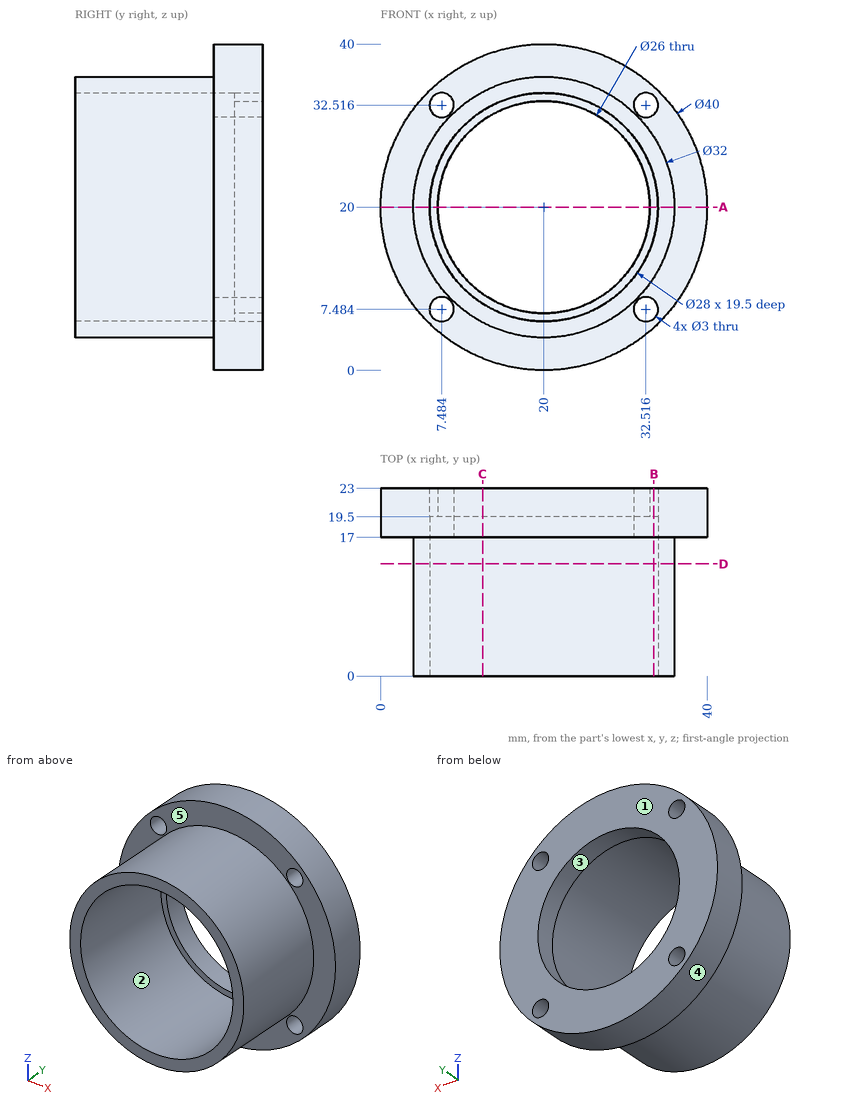
Drawing for the job (mm, zero at the part's lowest x, y, z). A direction names the side the tool comes from. Give positions to 0.01 mm unless a question says otherwise; leave off trailing zeros. Order: outer loops, then holes, each group sorted by start corner. A loop starts at its lowest first (then second) coordinate and runs counter-clockwise, first axis right, second up. Notation, with made-up numbers: (-30.75, 39.5) - (5.25, 39.5) arc R22 ccw to (5.25, 69.5) - close; hole circle Ø3 at (-5, 2.5). An arc over 180 degrees is marked (long way). Use one line per item in the form item = value.
Item 1: Probe probe 1 along X at (y, z) = (22.15, 20); probe 2 along X at (y, z) = (8.25, 20); probe 3 along Y at (x, z) = (24, 32.5). List the from-to ranges inside material, lowest first. Write a range as from..to.
Solution:
probe_1 = 0..7, 33..40
probe_2 = 4..6, 34..36
probe_3 = 19.5..23
Item 2: Pin check, flat tips, straight feed: pin 1 Ø10 at (x, y) = (17, 12.5) entering from -Z; pin 2 Ø17 at (x, z) = (20, 20) entering from -Y; pin 3 Ø4 at (x, z) = (31, 26) entering from -Y; pin 4 Ø14 at (x, z) = (17.5, 13.5) entering from -Y. Stop position of each tip, or through.
Solution:
pin_1 = 0.02
pin_2 = through
pin_3 = 0
pin_4 = 19.5
Item 3: Two-plate mould, pull along Z, no slides. Class the marked faces 3, 4 and 5: released by +Z, released by -Z, zero draft, split by the parting line, or undercut.
Solution:
face_3 = undercut
face_4 = split by the parting line
face_5 = zero draft
Item 4: Slice it at A-A on z = 20. Give the cut face in (x, y), and give its area (3 significant figures).
Solution:
outline = (0, 17) - (4, 17) - (4, 0) - (6, 0) - (6, 19.5) - (7, 19.5) - (7, 23) - (0, 23) - close; (33, 19.5) - (34, 19.5) - (34, 0) - (36, 0) - (36, 17) - (40, 17) - (40, 23) - (33, 23) - close
area = 147 mm2
Item 5: Which spindle directions (+Z, -Z, +X, -X, +Y, -Y) get a long thin tool onto all of the face, cutting with end or side? Do the marked faces 1 and 2. Say none if no direction does.
Solution:
face_1 = +Z, -Z, +X, -X, +Y
face_2 = -Y
Item 6: Slice it at C-C on x = 12.5. Give the cut face in (y, z).
Solution:
outline = (0, 5.87) - (17, 5.87) - (17, 1.46) - (23, 1.46) - (23, 9.38) - (19.5, 9.38) - (19.5, 8.18) - (0, 8.18) - close; (0, 31.82) - (19.5, 31.82) - (19.5, 30.62) - (23, 30.62) - (23, 38.54) - (17, 38.54) - (17, 34.13) - (0, 34.13) - close
Item 7: Slice it at B-B on x = 33.5. Give the cut face in (y, z).
Solution:
outline = (0, 11.41) - (17, 11.41) - (17, 8.62) - (23, 8.62) - (23, 31.38) - (17, 31.38) - (17, 28.59) - (0, 28.59) - (0, 23.71) - (19.5, 23.71) - (19.5, 16.29) - (0, 16.29) - close; (17, 5.24) - (23, 5.24) - (23, 6.35) - (17, 6.35) - close; (17, 33.65) - (23, 33.65) - (23, 34.76) - (17, 34.76) - close
Item 8: Slice it at D-D on y = 13.75. Give the cut face in (x, z).
Solution:
outline = circle Ø32 at (20, 20); hole circle Ø28 at (20, 20)
